Autodesk Inventor part; units mm, degrees
ref_plane "YZ Plane" through (0, 0, 0) normal (1, 0, 0) x (0, 1, 0)
ref_plane "XZ Plane" through (0, 0, 0) normal (0, 1, 0) x (-1, 0, 0)
ref_plane "XY Plane" through (0, 0, 0) normal (0, 0, 1) x (1, 0, 0)
sketch "Sketch1" plane through (0, 0, 0) normal (0, 0, 1) x (1, 0, 0)
  circle A0 centre (0, 0) radius 7.5
  dimension "d0" = 15
extrude "Extrusion1" add sketch "Sketch1" along normal blind 5
sketch "Sketch2" plane through (0, 0, 0) normal (0, 0, -1) x (-1, 0, 0)
  circle A0 centre (0, 0) radius 6.5
  circle A1 centre (0, 0) radius 5
  circle A2 centre (0, 0) radius 7.5
  dimension "d3" = 13
  dimension "d4" = 15
  dimension "d5" = 10
extrude "Extrusion2" add sketch "Sketch2" along normal blind 2 contours A0
sketch "Sketch3" plane through (0, 0, 5) normal (0, 0, 1) x (1, 0, 0)
  circle A0 centre (0, 0) radius 7.5
  circle A1 centre (0, 0) radius 2.5
  dimension "d8" = 15
  dimension "d13" = 5
extrude "Extrusion3" add sketch "Sketch3" along normal blind 5 contours A1
chamfer "Chamfer1" distance 2 angle 68.199 1 edges at (5, 0, 0) measured on face at (-4.9838, -0.4023, -1.3333)
properties part number "stredne_koleso"
Can you work these out from the model? Positions are in its coordinate system, mm. A direction names the side the tool comes from. Coordinates: 2 decimals unless noted, no trailing zeros. Loops run counter-clockwise (first coordinate to the right, second up) from the corner with the lowest first, then second, coordinate; pieces in that order, holes last. Notation, with made-up numbers: (66.25, -23.75) - (84.25, -23.75) arc R16 ccw to (84.25, 3.25) - close; hole circle Ø3 at (38, 71.25). An arc over 180 degrees is marked (long way). Use a Markdown table: item, result.
Item 1: We'd pull the mould along X, two halves only. Please class faces 1 (the face through (-0.54, 2.44, 7.46)), 2 (the face through (-0.299, 0.094, -0.125)), 3 (the face through (-6, 3, 0)): released by +X, released by -X, zero draft, split by the parting line, or undercut.
Numbers:
| item | result |
|---|---|
| face 1 | split by the parting line |
| face 2 | undercut |
| face 3 | zero draft |
Item 2: For faces 4 (the face through (5.158, 3.955, -0.986)), 5 (the face through (-2, 2, 5)), 6 (the face through (-2, -5, -2)), which set-ups out of +Z, -Z, +X, -X, +Y, -Y let a thin tool reach every point of the face, with its end or its side?
Numbers:
| item | result |
|---|---|
| face 4 | -Z |
| face 5 | +Z |
| face 6 | -Z, +X, -X, +Y, -Y |
Item 3: I want a section at D-D on z = 3.5. Please give me the cut outline in (x, y), and give its area (3 significant figures).
Numbers:
| item | result |
|---|---|
| outline | circle Ø15 at (0, 0) |
| area | 177 mm2 |
Item 4: If I drill on probe 1 along Z at (x, y) = (-1, 6.5); probe 2 along Z at (x, y) = (0.5, -5.75); probe 3 along Y at (x, z) = (6, -1), over which ranges is the centre line in solid material (lowest first)? Write a range as from..to.
Numbers:
| item | result |
|---|---|
| probe 1 | z = 0..5 |
| probe 2 | z = -2..5 |
| probe 3 | y = -2.5..2.5 |
Item 5: I want a section at C-C on y = 5.5. Please give me the cut outline in (x, z).
Numbers:
| item | result |
|---|---|
| outline | (-5.1, 0) - (-3.46, 0) - (-3.46, -2) - (3.46, -2) - (3.46, 0) - (5.1, 0) - (5.1, 5) - (-5.1, 5) - close |
Item 6: I want a section at A-A on z = 8.5. Please give me the cut outline in (x, y).
Numbers:
| item | result |
|---|---|
| outline | circle Ø5 at (0, 0) |
Item 7: Will these pins go through, and if not, where does the flat tip stop? pin 1 (6 mm diameter, centred on x = -3, z = -1, fed in from +Y); pin 2 (6 mm diameter, centred on x = 0, y = 0, fed in from -Z); pin 3 (1.5 mm diameter, centred on x = -1, y = 2.5, fed in from -Z); pin 4 (4 mm diameter, centred on y = -2, z = 0.5, fed in from -X).
Numbers:
| item | result |
|---|---|
| pin 1 | stops at y = 7.5 |
| pin 2 | stops at z = -1.2 |
| pin 3 | stops at z = -1.38 |
| pin 4 | stops at x = -7.5 |
Item 8: I want a section at B-B on x = 5.75. Please give me the cut outline in (y, z), and give its area (3 significant figures).
Numbers:
| item | result |
|---|---|
| outline | (-4.82, 0) - (-3.03, 0) - (-3.03, -2) - (3.03, -2) - (3.03, 0) - (4.82, 0) - (4.82, 5) - (-4.82, 5) - close |
| area | 60.3 mm2 |
